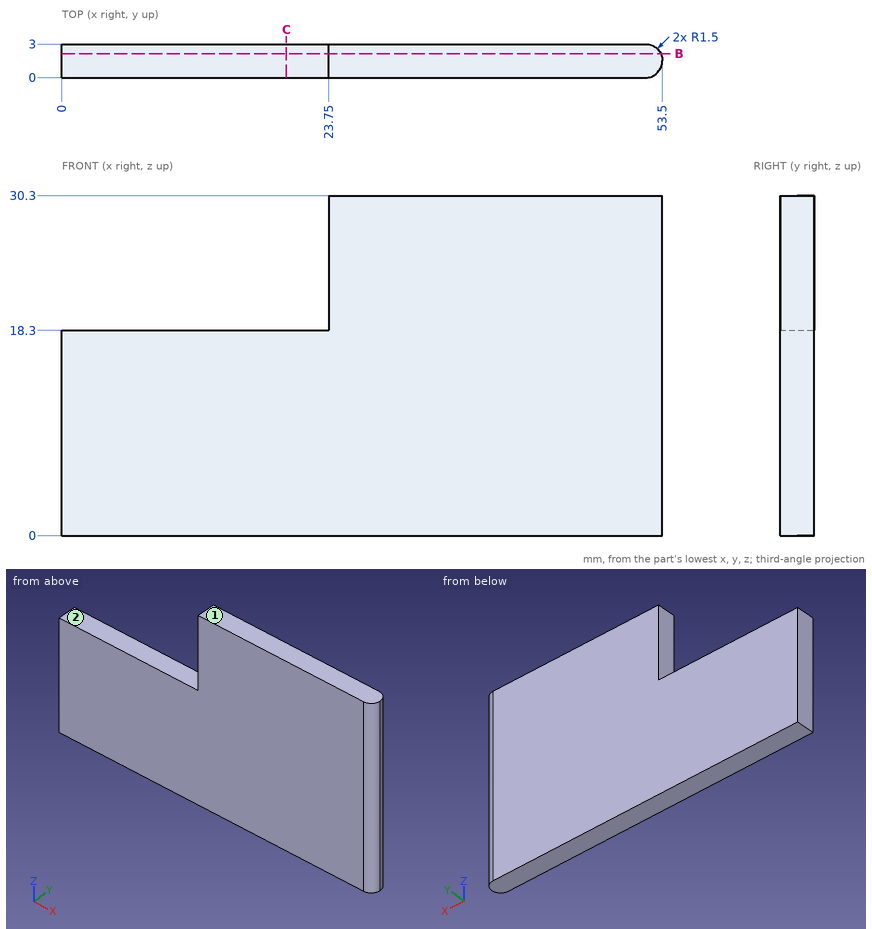
Can you work these out from the drawing? Everything is in mm from the part's minimum corner. A direction names the side the tool comes from. Coordinates: 2 decimals unless noted, no trailing zeros. Loops run counter-clockwise (first coordinate to the right, second up) from the corner with the lowest first, then second, coordinate; pieces in that order, holes last. Notation, with made-up numbers: (-13.75, 67) - (15.25, 67) arc R34 ccw to (15.25, 102) - close; hole circle Ø11 at (-23.5, 53). An arc over 180 degrees is marked (long way). Answer as CSV lines item,"result".
Q1. If I drill on L1, parallel to X at y = 1.5, z = 22.5; L2, parallel to X at y = 1.4, z = 10; L3, parallel to Z at x = 16, y = 1.65, over which ranges is the centre line in solid material (lowest first)? Write a range as [from, to].
Response:
L1,"[23.75, 53.5]"
L2,"[0, 53.5]"
L3,"[0, 18.3]"
Q2. If we section it at B-B, the plane y = 2.15: Write out the boundary of the cut face in (x, z), and give its area (3 significant figures).
Response:
outline,"(0, 0) - (53.35, 0) - (53.35, 30.3) - (23.75, 30.3) - (23.75, 18.3) - (0, 18.3) - close"
area,"1,330 mm2"
Q3. For pin 1 (0.9 mm diameter, centred on x = 14.5, y = 1, fed in from +Z), with a flat end and sliding along its axis, tell me the tip position at first contact or that it passes through.
Response:
pin 1,"z = 18.3"
Q4. If we section it at C-C, the plane x = 20: Write out the boundary of the cut face in (y, z), and give its area (3 significant figures).
Response:
outline,"(0, 0) - (3, 0) - (3, 18.3) - (0, 18.3) - close"
area,"54.9 mm2"
Q5. For the marked faces 1 and 2, which set-ups out of +Z, -Z, +X, -X, +Y, -Y let a thin tool reach every point of the face, with its end or its side?
Response:
face 1,"+Z, +X, -X, +Y, -Y"
face 2,"+Z, -X, +Y, -Y"
